Verification items for this drawing (mm, ordinates from the low corner). A direction names the side the tool comes from. Give positions to 0.01 mm unless a question says otherwise; leave off trailing zeros. Order: outer loops, then holes, each group sorted by start corner. A loop starts at its lowest first (then second) coordinate and runs counter-clockwise, first axis right, second up. Notation, with made-up numbers: M 20,-15.75 L 64,-15.75 A31 cw 64,10.25 Z; hole C -32,-3.5 d4. An arc over 180 degrees is marked long. One line per question, with ' | ' between items. Start each with the question number.
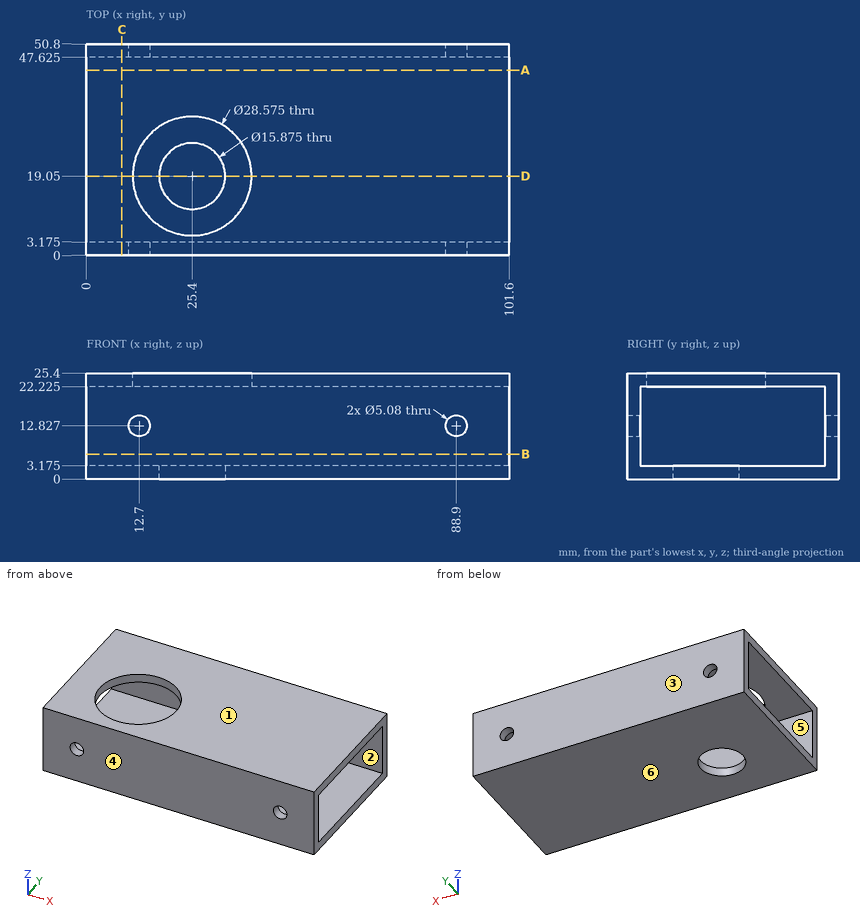
Item 1: Cross-section at D-D, the plane y = 19.05. Record the cut outline in (x, z) (1 decimal), plus the area to 3 significant figures.
Item 2: Set-up check for the marked faces 5 and 6: record each of +Z, -Z, +X, -X, +Y, -Y from which the full face is reachable in a straight line by a thin tool's end or side.
Item 3: Cross-section at C-C, the plane x = 8.5. Record the cut outline in (y, z) (3 decimals), plus the area to 3 significant figures.
Item 4: Material ranges on line 1 along Y through (x, z) = (50.5, 10.75) (3 decimals); line 2 along Z through (x, y) = (34, 44.5) (3 decimals); line 3 along Z through (x, y) = (12.7, 49.7), recorded low to high.
Item 5: Mould release check, pull along Y, two halves, no side actions. Record for the marked faces 1, 2, 3 and 4: released by +Y, released by -Y, zero draft, split by the parting line, or undercut.
Item 6: Cross-section at B-B, the plane z = 6. Record the cut outline in (x, y) (3 decimals).
Item 7: Cross-section at A-A, the plane y = 44.5. Record the cut outline in (x, z) (3 decimals).
Outcome:
1) outline: M 0,0 L 17.5,0 L 17.5,3.2 L 0,3.2 Z; M 0,22.2 L 11.1,22.2 L 11.1,25.4 L 0,25.4 Z; M 33.3,0 L 101.6,0 L 101.6,3.2 L 33.3,3.2 Z; M 39.7,22.2 L 101.6,22.2 L 101.6,25.4 L 39.7,25.4 Z | area: 504 mm²
2) face 5: +X, -X | face 6: -Z, +X, -X, +Y, -Y
3) outline: M 0,0 L 50.8,0 L 50.8,25.4 L 0,25.4 Z; hole M 3.175,3.175 L 47.625,3.175 L 47.625,22.225 L 3.175,22.225 Z | area: 444 mm²
4) line 1: y = 0 to 3.175, 47.625 to 50.8 | line 2: z = 0 to 3.175, 22.225 to 25.4 | line 3: z = 0 to 10.29, 15.37 to 25.4
5) face 1: zero draft | face 2: undercut | face 3: released by +Y | face 4: released by -Y
6) outline: M 0,0 L 101.6,0 L 101.6,3.175 L 0,3.175 Z; M 0,47.625 L 101.6,47.625 L 101.6,50.8 L 0,50.8 Z
7) outline: M 0,0 L 101.6,0 L 101.6,3.175 L 0,3.175 Z; M 0,22.225 L 101.6,22.225 L 101.6,25.4 L 0,25.4 Z
